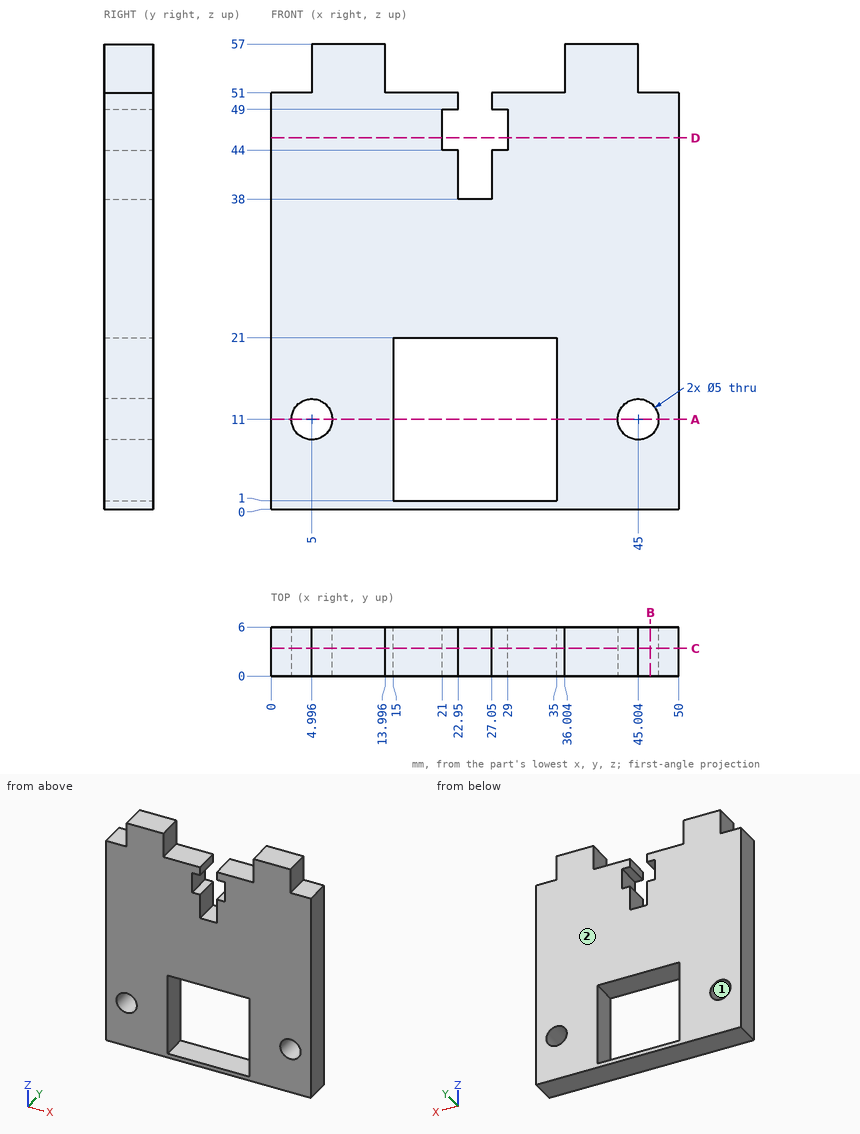
Print and shaded views of the part. All mm, measured from the part's lowest x, y and z. Coordinates: 2 decimals unless noted, no trailing zeros. Order: outer loops, then holes, each group sorted by start corner. A loop starts at its lowest first (then second) coordinate and runs counter-clockwise, first axis right, second up.
(1) Slice it at A-A, the plane z = 11. Write the cut outline in (x, y).
Check sheet entries:
outline: (0, 0) - (2.5, 0) - (2.5, 6) - (0, 6) - close; (7.5, 0) - (15, 0) - (15, 6) - (7.5, 6) - close; (35, 0) - (42.5, 0) - (42.5, 6) - (35, 6) - close; (47.5, 0) - (50, 0) - (50, 6) - (47.5, 6) - close
(2) Slice it at B-B, the plane x = 46.5. Write the cut outline in (y, z).
Check sheet entries:
outline: (0, 0) - (6, 0) - (6, 9) - (0, 9) - close; (0, 13) - (6, 13) - (6, 51) - (0, 51) - close
(3) Slice it at C-C, the plane y = 3.4. State how many separate pieces and enclosed holes the cut face has, and give its area (3 significant figures).
Check sheet entries:
separate pieces: 1
enclosed holes: 3
area: 2,150 mm2
(4) Pull direction X, two halves, no side cores. Call the marked faces 1 and 2: pulls with the +X half, pulls with the -X half, needs draft (parallel to the pull), parting line crosses it, or undercut.
Check sheet entries:
face 1: undercut
face 2: needs draft
(5) Slice it at D-D, the plane z = 45.5. Write the cut outline in (x, y).
Check sheet entries:
outline: (0, 0) - (21, 0) - (21, 6) - (0, 6) - close; (29, 0) - (50, 0) - (50, 6) - (29, 6) - close
(6) Probe L1, parallel to Z at x = 22, y = 4.9; L2, parallel to X at y = 4.2, z = 42.5; L3, parallel to X at y = 3.95, z = 45. List the from-to ranges inside material, lowest first.
Check sheet entries:
L1: z = 0 to 1, 21 to 44, 49 to 51
L2: x = 0 to 22.95, 27.05 to 50
L3: x = 0 to 21, 29 to 50
(7) Pin check, flat tips, straight feed: pin 1 Ø1.8 at (x, y) = (30.5, 3.5) entering from +Z; pin 2 Ø3 at (y, z) = (2, 53) entering from +X. Stop position of each tip, or through.
Check sheet entries:
pin 1: stops at z = 51
pin 2: stops at x = 45
